For this review, take the finished solid that the model builds, in its own axes (mm). Give positions to 0.01 mm unless a question says otherwise; leave off trailing zeros. Loops run counter-clockwise (first coordinate to the right, second up) from the corner with the lowest first, then second, coordinate; pieces in that order, holes last.
```python
from build123d import *

# Parameters (mm, degrees)
SKETCH1_R           = 2.25
BOSS_EXTRUDE1_DEPTH = 64
SKETCH1_3_R         = 1.375
BOSS_EXTRUDE2_DEPTH = 1
SKETCH5_R           = 1.25
BOSS_EXTRUDE3_DEPTH = 1
SKETCH6_R           = 2
BOSS_EXTRUDE4_DEPTH = 1
SKETCH12_R          = 1.4
CUT_EXTRUDE1_DEPTH  = 7.5


with BuildPart() as part:
    # Sketch1 → Boss-Extrude1 (new body)
    with BuildSketch(Plane(origin=(0, 0, 0), x_dir=(1, 0, 0), z_dir=(0, 1, 0))):
        with Locations((-0.522013312, 0.511138034)):
            Circle(SKETCH1_R)
    extrude(amount=BOSS_EXTRUDE1_DEPTH)

    # Sketch1<3> → Boss-Extrude2 (add)
    with BuildSketch(Plane(origin=(0, 0, 0), x_dir=(1, 0, 0), z_dir=(0, 1, 0))):
        with Locations((-0.522013312, 0.511138034)):
            Circle(SKETCH1_3_R)
    extrude(amount=BOSS_EXTRUDE2_DEPTH)

    # Sketch5 → Boss-Extrude3 (add)
    with BuildSketch(Plane.XZ):
        with Locations((-0.522013312, -0.511138034)):
            Circle(SKETCH5_R)
    extrude(amount=BOSS_EXTRUDE3_DEPTH)

    # Sketch6 → Boss-Extrude4 (add)
    with BuildSketch(Plane.XZ.offset(1)):
        with Locations((-0.522013312, -0.511138034)):
            Circle(SKETCH6_R)
    extrude(amount=BOSS_EXTRUDE4_DEPTH)

    # Sketch12 → Cut-Extrude1 (cut)
    with BuildSketch(Plane(origin=(0, 64, 0), x_dir=(1, 0, 0), z_dir=(0, 1, 0))):
        with Locations((-0.522013312, 0.511138034)):
            Circle(SKETCH12_R)
    extrude(amount=-CUT_EXTRUDE1_DEPTH, mode=Mode.SUBTRACT)


solid = part.part
```
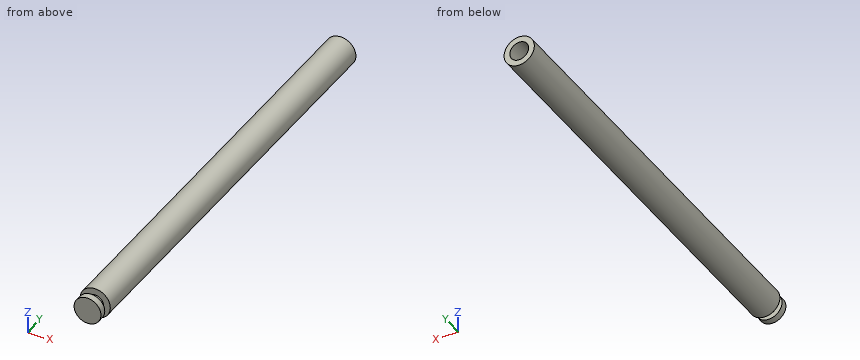
Q1. Consider section D-D on y = 60. Give the boundary of the cut face in (x, z), plus the area to 3 significant figures.
Answers:
outline: circle Ø4.5 at (-0.52, -0.51); hole circle Ø2.8 at (-0.52, -0.51)
area: 9.75 mm2
Q2. For probe 1 along Y at (x, z) = (1, -0.05); probe 2 along X at (y, z) = (45, -0.4); probe 3 along Y at (x, z) = (-0.05, -0.1), list the stretches that pass through material, from the lowest coordinate up.
Answers:
probe 1: y = -2 to -1, 0 to 64
probe 2: x = -2.77 to 1.73
probe 3: y = -2 to 56.5
Q3. Consider section C-C on y = 26.5. Give the boundary of the cut face in (x, z).
Answers:
outline: circle Ø4.5 at (-0.52, -0.51)
Q4. Consider section B-B on x = -0.35. Give the boundary of the cut face in (y, z), plus the area to 3 significant figures.
Answers:
outline: (-2, -2.5) - (-1, -2.5) - (-1, -1.75) - (0, -1.75) - (0, -2.75) - (64, -2.75) - (64, -1.9) - (56.5, -1.9) - (56.5, 0.88) - (64, 0.88) - (64, 1.73) - (0, 1.73) - (0, 0.73) - (-1, 0.73) - (-1, 1.48) - (-2, 1.48) - close
area: 273 mm2
Q5. For pin 1 Ø1 at (y, z) = (5, -1.5) entering from +X; pin 2 Ø1.4 at (x, z) = (-0.5, -0.5) entering from +Y, all flat-tipped, find the tip position at first contact; note any pin that passes through.
Answers:
pin 1: stops at x = 1.67
pin 2: stops at y = 56.5
Q6. Consider section A-A on z = 0.1. Give the boundary of the cut face in (x, y), plus the area to 3 significant figures.
Answers:
outline: (-2.69, 0) - (-1.61, 0) - (-1.61, -1) - (-2.43, -1) - (-2.43, -2) - (1.38, -2) - (1.38, -1) - (0.57, -1) - (0.57, 0) - (1.64, 0) - (1.64, 64) - (0.74, 64) - (0.74, 56.5) - (-1.78, 56.5) - (-1.78, 64) - (-2.69, 64) - close
area: 264 mm2
